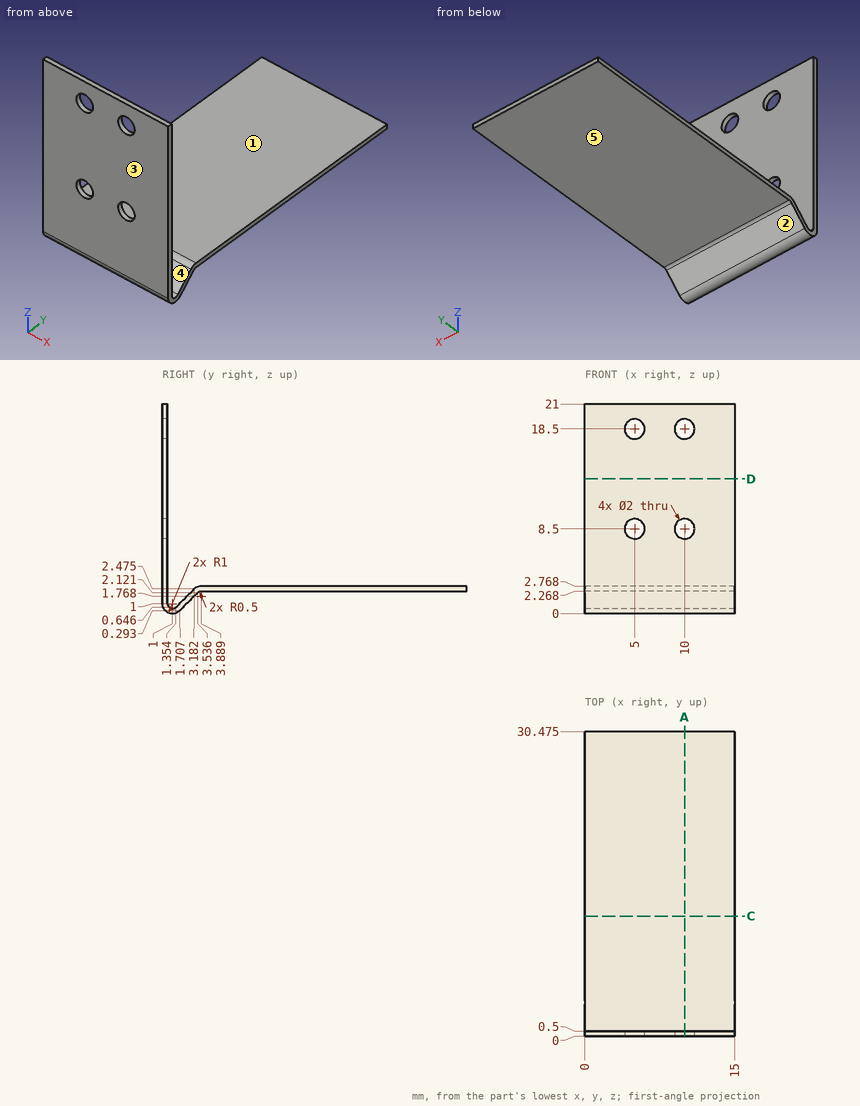
The drawing under review shows one solid part. Ordinate dimensions are in mm from its lowest x, y, z. A direction names the side the tool comes from. Coordinates: 2 decimals unless noted, no trailing zeros. Order: outer loops, then holes, each group sorted by start corner. A loop starts at its lowest first (then second) coordinate and runs counter-clockwise, first axis right, second up. Notation, with made-up numbers: (72.5, 4.5) -> (99.5, 4.5) arc R19 ccw to (99.5, 29.5) -> close; hole circle Ø6 at (78.25, 4.5). An arc over 180 degrees is marked (long way). Use CSV: the item, a comma, the result in double quotes. Start each with the question number.
Item 1: Wall thickness on probe 1 along Z at (x, y) = (5, 0.3) (1 decimal); probe 2 along Z at (x, y) = (10, 0.35); probe 3 along Y at (x, z) = (6, 3.25): over which ranges is each line inside the solid? List them lowest first.
Item 2: Draft analysis for pull direction Y (two halves, no side actions). For the marked faces 3, 4 and 5, state which applies: pulls with the +Y half, pulls with the -Y half, needs draft (parallel to the pull), parting line crosses it, or undercut.
Item 3: We need section C-C, the plane y = 12. Give the boundary of the cut face in (x, z).
Item 4: For the marked faces 1 and 2, list the 3-axis set-ups (+Z, -Z, +X, -X, +Y, -Y) from which the entire face can be reached by the end or side of a thin tool; tool diameter is ignored.
Item 5: We need section A-A, the plane x = 10. Give the number of separate pieces and of enclosed holes in the cut face.
Item 6: We need section D-D, the plane z = 13.5. Give the boundary of the cut face in (x, y).
Item 7: Insertion check: pin 1 (2.5 mm diameter, centred on x = 10, z = 8.5, fed in from -Y); pin 2 (7.5 mm diameter, centred on x = 6, y = 12.5, fed in from +Z); pin 3 (1.5 mm diameter, centred on x = 1.5, z = 12, fed in from +Y); pin 4 (7.5 mm diameter, centred on x = 4.5, y = 19, fed in from -Z). Each pin has a flat end and moves straight along its axis. Give the tip position at first contact, or say it passes through.
Derived:
1,probe 1,"z = 0.3 to 7.5, 9.5 to 17.5, 19.5 to 21"
1,probe 2,"z = 0.24 to 7.5, 9.5 to 17.5, 19.5 to 21"
1,probe 3,"y = 0 to 0.5"
2,face 3,"pulls with the -Y half"
2,face 4,"undercut"
2,face 5,"needs draft"
3,outline,"(0, 2.27) -> (15, 2.27) -> (15, 2.77) -> (0, 2.77) -> close"
4,face 1,"+Z, +X, -X, +Y"
4,face 2,"-Z, +X, -X, +Y"
5,separate pieces,"3"
5,enclosed holes,"0"
6,outline,"(0, 0) -> (15, 0) -> (15, 0.5) -> (0, 0.5) -> close"
7,pin 1,"stops at y = 0"
7,pin 2,"stops at z = 2.77"
7,pin 3,"stops at y = 0.5"
7,pin 4,"stops at z = 2.27"
